```python
from build123d import *

# Parameters (mm, degrees)
F1_DEPTH = 25.4
F2_R     = 2.921
F2_R_2   = 1.778
F3_DEPTH = 25.4
F4_DEPTH = 1.27
F5_W     = 36.3684481568
F5_H     = 3.302
F6_DEPTH = 1.524
F8_DEPTH = 2.54


with BuildPart() as f1:
    # F0 (on Front) → F1 (new body)
    with BuildSketch(Plane.XZ):
        Polygon((16.5742833321, 18.1842240784), (-14.9217166679, 0), (16.5742833321, 0), align=None)
    extrude(amount=F1_DEPTH)

    # F2 (on face) → F3 (cut)
    with BuildSketch(Plane(origin=(0, 0, 0), x_dir=(1, 0, 0), z_dir=(0, 0, -1))):
        with Locations((-7.0477166679, 19.05)):
            Circle(F2_R)
        with Locations((-7.0477166679, 19.05)):
            Circle(F2_R_2, mode=Mode.SUBTRACT)
        with Locations((8.7002833321, 19.05)):
            Circle(F2_R)
        with Locations((8.7002833321, 19.05)):
            Circle(F2_R_2, mode=Mode.SUBTRACT)
        with Locations((-7.0477166679, 6.35)):
            Circle(F2_R)
        with Locations((-7.0477166679, 6.35)):
            Circle(F2_R_2, mode=Mode.SUBTRACT)
        with Locations((8.7002833321, 6.35)):
            Circle(F2_R)
        with Locations((8.7002833321, 6.35)):
            Circle(F2_R_2, mode=Mode.SUBTRACT)
        with Locations((-7.0477166679, 19.05)):
            Circle(F2_R_2)
        with Locations((8.7002833321, 19.05)):
            Circle(F2_R_2)
        with Locations((-7.0477166679, 6.35)):
            Circle(F2_R_2)
        with Locations((8.7002833321, 6.35)):
            Circle(F2_R_2)
    extrude(amount=-F3_DEPTH, mode=Mode.SUBTRACT)

    # F2 (on face) → F4 (join)
    with BuildSketch(Plane(origin=(0, 0, 0), x_dir=(1, 0, 0), z_dir=(0, 0, -1))):
        with Locations((-7.0477166679, 19.05)):
            Circle(F2_R)
        with Locations((-7.0477166679, 19.05)):
            Circle(F2_R_2, mode=Mode.SUBTRACT)
        with Locations((8.7002833321, 19.05)):
            Circle(F2_R)
        with Locations((8.7002833321, 19.05)):
            Circle(F2_R_2, mode=Mode.SUBTRACT)
        with Locations((-7.0477166679, 6.35)):
            Circle(F2_R)
        with Locations((-7.0477166679, 6.35)):
            Circle(F2_R_2, mode=Mode.SUBTRACT)
        with Locations((8.7002833321, 6.35)):
            Circle(F2_R)
        with Locations((8.7002833321, 6.35)):
            Circle(F2_R_2, mode=Mode.SUBTRACT)
    extrude(amount=-F4_DEPTH)

    # F5 (on face) → F6 (join)
    with BuildSketch(Plane(origin=(-3.730429167, 0, 6.4612928512), x_dir=(0.8660254038, 0, 0.5), z_dir=(-0.5, 0, 0.8660254038))):
        with Locations((5.2616383759, -12.7)):
            Rectangle(F5_W, F5_H)
    extrude(amount=F6_DEPTH)

    # F7 (on face) → F8 (join)
    with BuildSketch(Plane(origin=(-4.492429167, 0, 7.7811155666), x_dir=(0.8660254038, 0, 0.5), z_dir=(-0.5, 0, 0.8660254038))):
        Polygon((-12.9225857025, -10.287), (-12.9225857025, -12.7), (-12.9225857025, -15.113), (23.4458624543, -15.113), (23.4458624543, -12.7), (23.4458624543, -10.287), align=None)
    extrude(amount=F8_DEPTH)


solid = f1.part
```
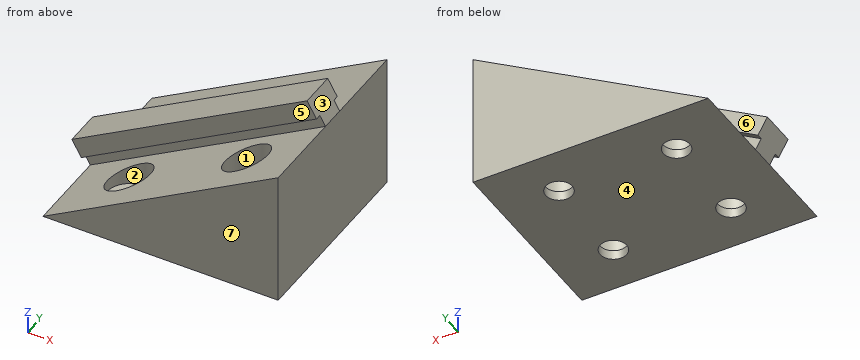
For this review, take the finished solid that the model builds, in its own axes (mm). Face numbers are marked on the shaded views. A direction names the side the tool comes from. Round coordinates to 2 decimals unless told otherwise and drop trailing zeros. Write each loop counter-clockwise with the first axis right and the second up, starting at its lowest first coordinate (ties: lowest second). Pieces come first, ordered by that corner, then holes. Notation, with made-up numbers: (-36, 44.5) - (21, 44.5) arc R12 cw to (21, 48.5) - close; hole circle Ø2 at (42, 52.5). An arc over 180 degrees is marked (long way). Write each question's results on one line, items separated by ' | '.
Item 1: For the marked faces 5, 6 and 7, list the 3-axis set-ups (+Z, -Z, +X, -X, +Y, -Y) from which the entire face can be reached by the end or side of a thin tool; tool diameter is ignored.
Calculated:
face 5: +Z, -X, -Y | face 6: +Z, -X, +Y | face 7: +Z, -Z, +X, -X, -Y
Item 2: Take a section at D-D on z = 2.5. State the section outline as (x, y) points, then the cut area to 3 significant figures.
Calculated:
outline: (-16.37, -15.11) - (-13.64, -15.11) - (-13.64, -14.35) - (-10.59, -14.35) - (-10.59, -25.4) - (16.57, -25.4) - (16.57, 0) - (-10.59, 0) - (-10.59, -11.05) - (-13.64, -11.05) - (-13.64, -10.29) - (-16.37, -10.29) - close; hole circle Ø5.84 at (-7.05, -19.05); hole circle Ø5.84 at (-7.05, -6.35); hole circle Ø5.84 at (8.7, -19.05); hole circle Ø5.84 at (8.7, -6.35) | area: 606 mm^2
Item 3: To check wall thickness, follow line 1 along X through (y, z) = (-6.35, 0.6); line 2 along X through (y, z) = (-6.35, 0.35); line 3 along X through (y, z) = (-19.05, 6). State the ranges of each line that lie inside material, in increasing order. Write a range as from..to.
Calculated:
line 1: x = -13.88..-8.83, -5.27..6.92, 10.48..16.57 | line 2: x = -14.32..-8.83, -5.27..6.92, 10.48..16.57 | line 3: x = -4.13..5.78, 11.62..16.57
Item 4: Take a section at B-B on z = 11.5. State the section outline as (x, y) points, then the cut area to 3 significant figures.
Calculated:
outline: (-3.13, -15.11) - (1.95, -15.11) - (1.95, -14.35) - (5, -14.35) - (5, -25.4) - (16.57, -25.4) - (16.57, 0) - (5, 0) - (5, -11.05) - (1.95, -11.05) - (1.95, -10.29) - (-3.13, -10.29) - close; hole circle Ø5.84 at (8.7, -19.05); hole circle Ø5.84 at (8.7, -6.35) | area: 275 mm^2
Item 5: For pin 1 (4.5 mm diameter, centred on x = 7.5, y = -19, fed in from +Z); pin 2 (5 mm diameter, centred on y = -7.5, z = 19.5, fed in from -X); pin 3 (1.5 mm diameter, centred on y = -21.5, z = 6.5, fed in from -X), all flat-tipped, find the tip position at first contact; note any pin that passes through.
Calculated:
pin 1: stops at z = 12.51 | pin 2: stops at x = 14.52 | pin 3: stops at x = -4.96
Item 6: Take a section at A-A on x = 8. State the section outline as (y, z) points.
Calculated:
outline: (-25.4, 0) - (-20.68, 0) - (-20.68, 1.27) - (-21.89, 1.27) - (-21.89, 13.23) - (-25.4, 13.23) - close; (-17.42, 0) - (-7.98, 0) - (-7.98, 1.27) - (-9.19, 1.27) - (-9.19, 13.23) - (-11.05, 13.23) - (-11.05, 14.99) - (-10.29, 14.99) - (-10.29, 17.93) - (-15.11, 17.93) - (-15.11, 14.99) - (-14.35, 14.99) - (-14.35, 13.23) - (-16.21, 13.23) - (-16.21, 1.27) - (-17.42, 1.27) - close; (-4.72, 0) - (0, 0) - (0, 13.23) - (-3.51, 13.23) - (-3.51, 1.27) - (-4.72, 1.27) - close
Item 7: Take a section at C-C on y = -6.35. State the section outline as (x, z) points, then the cut area to 3 significant figures.
Calculated:
outline: (-14.92, 0) - (-8.83, 0) - (-8.83, 1.27) - (-9.97, 1.27) - (-9.97, 2.86) - close; (-5.27, 0) - (6.92, 0) - (6.92, 1.27) - (5.78, 1.27) - (5.78, 11.95) - (-4.13, 6.23) - (-4.13, 1.27) - (-5.27, 1.27) - close; (10.48, 0) - (16.57, 0) - (16.57, 18.18) - (11.62, 15.32) - (11.62, 1.27) - (10.48, 1.27) - close | area: 186 mm^2
Item 8: Draft analysis for pull direction X (two halves, no side actions). For the marked faces 1, 2, 3 and 4, state which applies: pulls with the +X half, pulls with the -X half, needs draft (parallel to the pull), parting line crosses it, or undercut.
Calculated:
face 1: undercut | face 2: undercut | face 3: pulls with the +X half | face 4: needs draft
